Can you work these out from the model? Positions are in its coordinate system, mm. Face numbers are marked on the shaded views. Coordinates: 2 decimals unless noted, no trailing zeros. Order: outer loops, then holes, each group sorted by start corner. A loop starts at its lowest first (then second) coordinate and runs counter-clockwise, first axis right, second up. Notation, with made-up numbers: (-35, 85) -> (4, 85) arc R17 cw to (4, 98) -> close; hole circle Ø8 at (71.5, 79.25). An arc over 180 degrees is marked (long way). Use a Markdown table: item, result. Add a question column.
1. We'd pull the mould along Y, two halves only. Please class the marked faces 1, 2 and 3: pulls with the +Y half, pulls with the -Y half, needs draft (parallel to the pull), parting line crosses it, or undercut.
2. If I drill on line 1 along X through (y, z) = (10, 0.6); line 2 along Y through (x, z) = (-50, 1.35); line 3 along Y through (x, z) = (-50, 0.9), over which ranges is the centre line in solid material (lowest first)? Write a range as from..to.
3. Suppose I cut it at D-D, the plane x = -21.5. List the corners of the cut face in (y, z) for me, then the cut area to 3 significant figures.
4. For pin 1 Ø0.6 at (x, y) = (-81.5, 22) entering from -Z; pin 2 Ø2 at (x, z) = (-89, 15.5) entering from -Y; pin 3 Ø7 at (x, y) = (0, 10) entering from +Z, each with a flat end and sliding along its axis, tell me the tip position at first contact or that it passes through.
5. Suppose I cut it at C-C, the plane x = -55. List the corners of the cut face in (y, z) for me.
6. Suppose I cut it at B-B, the plane z = 9. List the corners of the cut face in (x, y) for me, then the cut area to 3 significant figures.
7. Suppose I cut it at A-A, the plane y = -10. List the corners of the cut face in (x, z) for me.
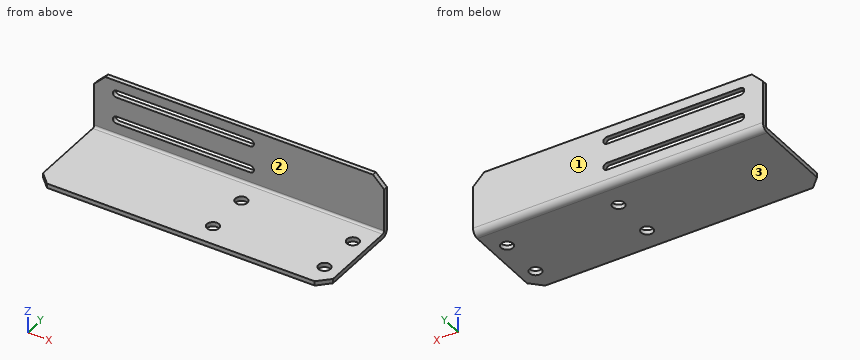
```python
from build123d import *

# Parameters (mm, degrees)
SKETCH_17_W             = 130
SKETCH_17_H             = 40
SM_BASE_FLANGE_1_DEPTH  = 2
HOLE_WIZARD_5_4_5_4_1_D = 5.4
SM_EDGE_FLANGE_1_DEPTH  = 130
CUT_EXTRUDE_4_REACH     = 135.822
CHAMFER_1_SIZE          = 5


# Sheet-metal steps are written as plain solids
with BuildPart() as part:
    # 草圖17 → 基材-凸緣1 (new body)
    with BuildSketch(Plane.XY):
        with Locations((-58, 0)):
            Rectangle(SKETCH_17_W, SKETCH_17_H)
    extrude(amount=SM_BASE_FLANGE_1_DEPTH)

    # Ø5.4 (5.4) 直徑孔1 (through all)
    with Locations(Plane(origin=(-278.067262353, 19.151419807, 2), x_dir=(-1, 0, 0), z_dir=(0, 0, 1))):
        with Locations((-228.067262353, 29.151419807), (-278.067262353, 29.151419807), (-228.067262353, 9.151419807), (-278.067262353, 9.151419807)):
            Hole(HOLE_WIZARD_5_4_5_4_1_D / 2)

    # 邊線-凸緣1 section (across the edge) → 邊線-凸緣1 (add)
    with BuildSketch(Plane(origin=(7, 21, 2), x_dir=(0, -1, 0), z_dir=(-1, 0, 0))):
        with BuildLine():
            Line((-2, 1), (-2, 25))
            Line((-2, 25), (0, 25))
            Line((0, 25), (0, 1))
            ThreePointArc((0, 1), (0.292893219, 0.292893219), (1, 0))
            Line((1, 0), (1, -2))
            ThreePointArc((1, -2), (-1.121320344, -1.121320344), (-2, 1))
        make_face()
    extrude(amount=SM_EDGE_FLANGE_1_DEPTH)

    # 草圖14 → 除料-伸長4 (cut, up to next)
    with BuildSketch(Plane(origin=(0, 23, 30.5), x_dir=(1, 0, 0), z_dir=(0, 1, 0)), mode=Mode.PRIVATE) as cut_extrude_4_sk1:
        with BuildLine():
            Line((-113, 19.9), (-53, 19.9))
            ThreePointArc((-53, 19.9), (-51.4, 21.5), (-53, 23.1))
            Line((-53, 23.1), (-113, 23.1))
            ThreePointArc((-113, 23.1), (-114.6, 21.5), (-113, 19.9))
        make_face()
    cut_extrude_4_tool1 = extrude(cut_extrude_4_sk1.sketch, amount=-CUT_EXTRUDE_4_REACH, mode=Mode.PRIVATE) & part.part
    # 草圖14 → 除料-伸長4 (cut, up to next)
    with BuildSketch(Plane(origin=(0, 23, 30.5), x_dir=(1, 0, 0), z_dir=(0, 1, 0)), mode=Mode.PRIVATE) as cut_extrude_4_sk2:
        with BuildLine():
            Line((-113, 7.9), (-53, 7.9))
            ThreePointArc((-53, 7.9), (-51.4, 9.5), (-53, 11.1))
            Line((-53, 11.1), (-113, 11.1))
            ThreePointArc((-113, 11.1), (-114.6, 9.5), (-113, 7.9))
        make_face()
    cut_extrude_4_tool2 = extrude(cut_extrude_4_sk2.sketch, amount=-CUT_EXTRUDE_4_REACH, mode=Mode.PRIVATE) & part.part
    add(cut_extrude_4_tool1.solids().sort_by_distance((-83, 23, 9))[0], mode=Mode.SUBTRACT)
    add(cut_extrude_4_tool2.solids().sort_by_distance((-83, 23, 21))[0], mode=Mode.SUBTRACT)

    # 導角1
    chamfer_1_edges = [part.edges().sort_by_distance(p)[0] for p in [
        (7, 22, 27),
        (-123, 22, 27),
        (7, -20, 1),
        (-123, -20, 1),
    ]]
    chamfer(chamfer_1_edges, length=CHAMFER_1_SIZE)


solid = part.part
```
Worked out:
| question | item | result |
|---|---|---|
| 1 | face 1 | pulls with the +Y half |
| 1 | face 2 | pulls with the -Y half |
| 1 | face 3 | needs draft |
| 2 | line 1 | x = -123..-52.7, -47.3..-2.7, 2.7..7 |
| 2 | line 2 | y = -20..-12.7, -7.3..7.3, 12.7..22.51 |
| 2 | line 3 | y = -20..-12.7, -7.3..7.3, 12.7..22.14 |
| 3 | outline | (-20, 0) -> (20, 0) arc R3 ccw to (23, 3) -> (23, 27) -> (21, 27) -> (21, 3) arc R1 cw to (20, 2) -> (-20, 2) -> close |
| 3 | area | 134 mm² |
| 4 | pin 1 | stops at z = 0.53 |
| 4 | pin 2 | stops at y = 21 |
| 4 | pin 3 | stops at z = 2 |
| 5 | outline | (-20, 0) -> (20, 0) arc R3 ccw to (23, 3) -> (23, 7.4) -> (21, 7.4) -> (21, 3) arc R1 cw to (20, 2) -> (-20, 2) -> close; (21, 10.6) -> (23, 10.6) -> (23, 19.4) -> (21, 19.4) -> close; (21, 22.6) -> (23, 22.6) -> (23, 27) -> (21, 27) -> close |
| 6 | outline | (-123, 21) -> (-114.6, 21) -> (-114.6, 23) -> (-123, 23) -> close; (-51.4, 21) -> (7, 21) -> (7, 23) -> (-51.4, 23) -> close |
| 6 | area | 134 mm² |
| 7 | outline | (-123, 0) -> (-52.7, 0) -> (-52.7, 2) -> (-123, 2) -> close; (-47.3, 0) -> (-2.7, 0) -> (-2.7, 2) -> (-47.3, 2) -> close; (2.7, 0) -> (7, 0) -> (7, 2) -> (2.7, 2) -> close |
